Verification items for the finished model (mm, model axes). Coordinates: 2 decimals unless noted, no trailing zeros. Order: outer loops, then holes, each group sorted by start corner. A loop starts at its lowest first (then second) coordinate and runs counter-clockwise, first axis right, second up. Notation, with made-up numbers: (47.25, 72.5) -> (62.25, 72.5) arc R4 ccw to (62.25, 77.5) -> close; hole circle Ø2 at (-26.75, 81.25). An arc over 180 degrees is marked (long way). Write item = value, one per line. Start each with the question number.
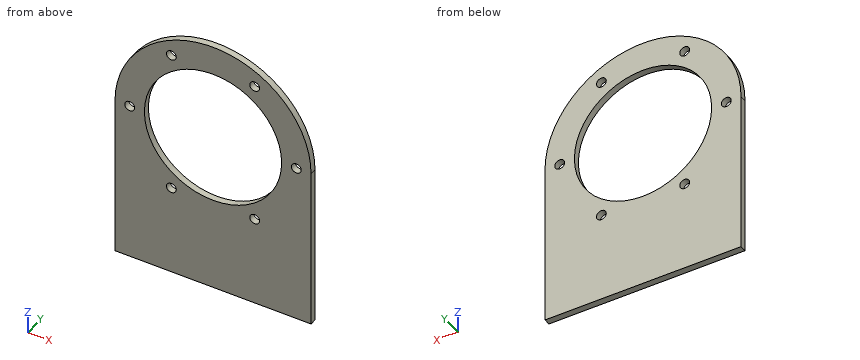
from build123d import *

# Parameters (mm, degrees)
SKETCH1_R           = 21
SKETCH1_R_2         = 1.5
BOSS_EXTRUDE1_DEPTH = 2


with BuildPart() as part:
    # Sketch1 → Boss-Extrude1 (new body)
    with BuildSketch(Plane(origin=(0, 0, 0), x_dir=(1, 0, 0), z_dir=(0, 1, 0))):
        with BuildLine():
            Line((-30, 0), (-30, 50))
            Line((-30, 50), (30, 50))
            Line((30, 50), (30, 0))
            ThreePointArc((30, 0), (0, -30), (-30, 0))
        make_face()
        with Locations(Location((0, 0, 0), (0, 0, 270))):
            Circle(SKETCH1_R, mode=Mode.SUBTRACT)
        with Locations(Location((-12.75, 22.083647797, 0), (0, 0, 270))):
            Circle(SKETCH1_R_2, mode=Mode.SUBTRACT)
        with Locations(Location((12.75, 22.083647797, 0), (0, 0, 270))):
            Circle(SKETCH1_R_2, mode=Mode.SUBTRACT)
        with Locations(Location((25.5, 0, 0), (0, 0, 270))):
            Circle(SKETCH1_R_2, mode=Mode.SUBTRACT)
        with Locations(Location((12.75, -22.083647797, 0), (0, 0, 270))):
            Circle(SKETCH1_R_2, mode=Mode.SUBTRACT)
        with Locations(Location((-12.75, -22.083647797, 0), (0, 0, 270))):
            Circle(SKETCH1_R_2, mode=Mode.SUBTRACT)
        with Locations(Location((-25.5, 0, 0), (0, 0, 270))):
            Circle(SKETCH1_R_2, mode=Mode.SUBTRACT)
    extrude(amount=BOSS_EXTRUDE1_DEPTH)


solid = part.part
Item 1: Section check B-B (y = 0.5). Record the boundary of the cut face in (x, z), then the cut area to 3 significant figures.
Item 2: Section check C-C (z = 6.5). Record the boundary of the cut face in (x, y), then the cut area to 3 significant figures.
Item 3: Thickness scan on line 1 (X direction, y = 0.35, z = 23); line 2 (X direction, y = 1.6, z = -23); line 3 (Z direction, x = 6, y = 0.85). Record the ranges inside material, lowest first.
Item 4: Section check A-A (x = 0). Record the boundary of the cut face in (y, z).
Item 5: Section check D-D (x = 12.75). Record the boundary of the cut face in (y, z), then the cut area to 3 significant figures.
Item 6: Gauge pin test, flat end, axial feed: P1, Ø2.5, axis at x = 12.75, z = -22.08, coming from the +Y side. Record the tip position at first contact, or that the pin passes through.
Filled sheet:
q1.outline = (-30, -50) -> (30, -50) -> (30, 0) arc R30 ccw to (-30, 0) -> close; hole circle Ø3 at (-25.5, 0); hole circle Ø42 at (0, 0); hole circle Ø3 at (-12.75, -22.08); hole circle Ø3 at (-12.75, 22.08); hole circle Ø3 at (12.75, -22.08); hole circle Ø3 at (12.75, 22.08); hole circle Ø3 at (25.5, 0)
q1.area = 2,990 mm^2
q2.outline = (-29.29, 0) -> (-19.97, 0) -> (-19.97, 2) -> (-29.29, 2) -> close; (19.97, 0) -> (29.29, 0) -> (29.29, 2) -> (19.97, 2) -> close
q2.area = 37.3 mm^2
q3.line_1 = -19.26 to -13.94, -11.56 to 11.56, 13.94 to 19.26
q3.line_2 = -30 to -13.94, -11.56 to 11.56, 13.94 to 30
q3.line_3 = -50 to -20.12, 20.12 to 29.39
q4.outline = (0, -50) -> (2, -50) -> (2, -21) -> (0, -21) -> close; (0, 21) -> (2, 21) -> (2, 30) -> (0, 30) -> close
q5.outline = (0, -50) -> (2, -50) -> (2, -23.58) -> (0, -23.58) -> close; (0, -20.58) -> (2, -20.58) -> (2, -16.69) -> (0, -16.69) -> close; (0, 16.69) -> (2, 16.69) -> (2, 20.58) -> (0, 20.58) -> close; (0, 23.58) -> (2, 23.58) -> (2, 27.16) -> (0, 27.16) -> close
q5.area = 75.6 mm^2
q6.P1 = through
